from build123d import *

# Parameters (mm, degrees)
SKETCH5_R          = 2.5
SKETCH5_R_2        = 12.5
CUT_EXTRUDE1_DEPTH = 10
SKETCH6_R          = 2.5
CUT_EXTRUDE2_DEPTH = 30
CIRPATTERN1_COUNT  = 5
CIRPATTERN1_ANGLE  = 150
CUT_EXTRUDE3_DEPTH = 2
SKETCH8_R          = 2.5
CUT_EXTRUDE4_DEPTH = 10
CIRPATTERN2_COUNT  = 45
CIRPATTERN2_ANGLE  = 180


with BuildPart() as part:
    # Sweep2: sweep along a path in Sketch4
    with BuildLine(Plane(origin=(0, 0, 0), x_dir=(0, 0, -1), z_dir=(1, 0, 0))) as sweep2_path:
        Line((0, 0), (-100, 0))
        ThreePointArc((-100, 0), (-400, 300), (-100, 600))
        Line((-100, 600), (0, 600))
    # Sketch2 → Sweep2 (sweep)
    with BuildSketch(Plane.XY):
        with BuildLine():
            Line((0, -44.5), (0, 44.5))
            ThreePointArc((0, 44.5), (-0.146446609, 44.853553391), (-0.5, 45))
            Line((-0.5, 45), (-29.5, 45))
            ThreePointArc((-29.5, 45), (-29.853553391, 44.853553391), (-30, 44.5))
            Line((-30, 44.5), (-30, 15))
            Line((-30, 15), (-28, 15))
            Line((-28, 15), (-28, 43))
            Line((-28, 43), (-2, 43))
            Line((-2, 43), (-2, -43))
            Line((-2, -43), (-28, -43))
            Line((-28, -43), (-28, -15))
            Line((-28, -15), (-30, -15))
            Line((-30, -15), (-30, -44.5))
            ThreePointArc((-30, -44.5), (-29.853553391, -44.853553391), (-29.5, -45))
            Line((-29.5, -45), (-0.5, -45))
            ThreePointArc((-0.5, -45), (-0.146446609, -44.853553391), (0, -44.5))
        make_face()
    sweep(path=sweep2_path.line)

    # Sketch5 → Cut-Extrude1 (cut)
    with BuildSketch(Plane(origin=(0, 0, 0), x_dir=(0, 0, -1), z_dir=(1, 0, 0))):
        with Locations((-78.991378029, 28.991378029)):
            Circle(SKETCH5_R)
        with Locations((-78.991378029, -28.991378029)):
            Circle(SKETCH5_R)
        with Locations((-21.008621971, 28.991378029)):
            Circle(SKETCH5_R)
        with Locations((-21.008621971, -28.991378029)):
            Circle(SKETCH5_R)
        with Locations((-65, 0)):
            Circle(SKETCH5_R_2)
    extrude(amount=-CUT_EXTRUDE1_DEPTH, mode=Mode.SUBTRACT)

    # Sketch6 → Cut-Extrude2 (cut)
    with BuildSketch(Plane.ZY.offset(30)):
        with Locations((169.881142178, 39.200026902)):
            Circle(SKETCH6_R)
        with Locations((185.410284884, -18.755522675)):
            Circle(SKETCH6_R)
    cut_extrude2 = extrude(amount=-CUT_EXTRUDE2_DEPTH, mode=Mode.SUBTRACT)

    # CirPattern1: Cut-Extrude2 ×5 about axis
    cirpattern1_axis = Axis((0, 300, 100), (-1, 0, 0))
    for i in range(1, CIRPATTERN1_COUNT):
        add(cut_extrude2.rotate(cirpattern1_axis, i * CIRPATTERN1_ANGLE / (CIRPATTERN1_COUNT - 1)), mode=Mode.SUBTRACT)

    # Sketch7 → Cut-Extrude3 (cut)
    with BuildSketch(Plane.ZY.offset(2)):
        with BuildLine():
            Line((75, 595.885896699), (25, 595.885896699))
            ThreePointArc((25, 595.885896699), (20, 600.885896699), (25, 605.885896699))
            Line((25, 605.885896699), (75, 605.885896699))
            ThreePointArc((75, 605.885896699), (80, 600.885896699), (75, 595.885896699))
        make_face()
    extrude(amount=-CUT_EXTRUDE3_DEPTH, mode=Mode.SUBTRACT)

    # Sketch8 → Cut-Extrude4 (cut)
    with BuildSketch(Plane.ZY.offset(2)):
        with Locations(Location((100, 0, 0), (0, 0, 90))):
            Circle(SKETCH8_R)
    cut_extrude4 = extrude(amount=-CUT_EXTRUDE4_DEPTH, mode=Mode.SUBTRACT)

    # CirPattern2: Cut-Extrude4 ×45 about axis
    cirpattern2_axis = Axis((0, 300, 100), (-1, 0, 0))
    for i in range(1, CIRPATTERN2_COUNT):
        add(cut_extrude4.rotate(cirpattern2_axis, i * CIRPATTERN2_ANGLE / (CIRPATTERN2_COUNT - 1)), mode=Mode.SUBTRACT)


solid = part.part
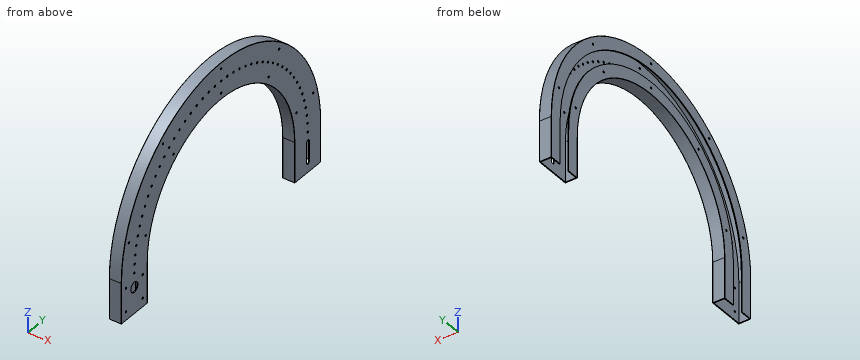
The listing builds one solid part. Answer for the finished solid, in the listing's coordinates (mm). Coordinates: 2 decimals unless noted, no trailing zeros. Write each loop counter-clockwise with the first axis right and the second up, starting at its lowest first coordinate (ties: lowest second). Pieces come first, ordered by that corner, then holes. Notation, with made-up numbers: (-2.5, 3) - (49.5, 3) arc R28 ccw to (49.5, 32) - close; hole circle Ø9 at (-21, 73). An arc over 180 degrees is marked (long way). Answer as CSV lines item,"result".
1. Find section A-A (x = -9). Give the vertices of the cut face in (y, z), plus the area to 3 significant figures.
Computed values:
outline,"(-45, 0) - (-43, 0) - (-43, 100) arc R343 cw to (643, 100) - (643, 0) - (645, 0) - (645, 100) arc R345 ccw to (-45, 100) - close; (43, 0) - (45, 0) - (45, 100) arc R255 cw to (555, 100) - (555, 0) - (557, 0) - (557, 100) arc R257 ccw to (43, 100) - close"
area,"4,570 mm²"
2. Find section B-B (z = 65). Give the number of separate pieces and of enclosed holes in the cut face, plus the area to 3 significant figures.
Computed values:
separate pieces,"4"
enclosed holes,"0"
area,"738 mm²"
3. Straight lines are drawn through the part: line 1 (Y direction, x = -27.5, z = 18); line 2 (X direction, y = 459, z = 302); line 3 (Y direction, x = -8, z = 106.5). For each, find the intervals that lie inside material, in ascending order. Write a range as [from, to].
Computed values:
line 1,"y = [-45, -43], [43, 45], [555, 557], [643, 645]"
line 2,"x = [-30, -28], [-2, 0]"
line 3,"y = [-44.94, -42.94], [43.08, 45.08], [554.92, 556.92], [642.94, 644.94]"
4. Given P1, Ø3, axis at y = 120.22, z = 340.16, coming from the +X side; P2, Ø6, axis at y = 236.23, z = 393.14, coming from the -X side; P3, Ø10, axis at x = -5, y = 202, coming from the -Z side; P4, Ø4, axis at x = -4.5, z = 333.5, coming from the -Y side, each flat-ended and moving along its own axis, determine where each tip first touches the part or whether it passes through.
Computed values:
P1,"passes through"
P2,"stops at x = -2"
P3,"stops at z = 333.27"
P4,"stops at y = 44.2"
